Here's how the part is built. I have some questions about the finished solid (model axes, mm). A direction names the side the tool comes from. Round coordinates to 2 decimals unless told otherwise and drop trailing zeros. Order: outer loops, then holes, each group sorted by start corner. A loop starts at its lowest first (then second) coordinate and runs counter-clockwise, first axis right, second up. Notation, with made-up numbers: (56, -33) -> (99, -33) arc R29 ccw to (99, 1) -> close; hole circle Ø7 at (39, 67). An arc over 180 degrees is marked (long way). Answer in a Markdown table with one row per item.
```python
from build123d import *

# Parameters (mm, degrees)
SKETCH_W        = 30
SKETCH_H        = 30
PAD_DEPTH       = 3
POCKET_DEPTH    = 2.5
SKETCH002_R     = 1.725
POCKET001_DEPTH = 5
SKETCH003_R     = 1.225
PAD001_DEPTH    = 1.5


with BuildPart() as part:
    # Sketch → Pad (new body)
    with BuildSketch(Plane.XZ):
        Rectangle(SKETCH_W, SKETCH_H)
    extrude(amount=-PAD_DEPTH)

    # Sketch001 (on Face6 of Pad) → Pocket (cut)
    with BuildSketch(Plane(origin=(0, 3, 0), x_dir=(1, 0, 0), z_dir=(0, 1, 0))):
        Polygon((-11.616581, 7.2), (-8.383419, 7.2), (-6.766838, 10), (-8.383419, 12.8), (-11.616581, 12.8), (-13.233162, 10), align=None)
        Polygon((11.616581, 7.2), (13.233162, 10), (11.616581, 12.8), (8.383419, 12.8), (6.766838, 10), (8.383419, 7.2), align=None)
        Polygon((11.616581, -12.8), (13.233162, -10), (11.616581, -7.2), (8.383419, -7.2), (6.766838, -10), (8.383419, -12.8), align=None)
        Polygon((-8.383419, -7.2), (-11.616581, -7.2), (-13.233162, -10), (-11.616581, -12.8), (-8.383419, -12.8), (-6.766838, -10), align=None)
    extrude(amount=-POCKET_DEPTH, mode=Mode.SUBTRACT)

    # Sketch002 (on Face33 of Pocket) → Pocket001 (cut)
    with BuildSketch(Plane(origin=(0, 0.5, 0), x_dir=(1, 0, 0), z_dir=(0, 1, 0))):
        with Locations((-10, 10)):
            Circle(SKETCH002_R)
        with Locations((10, 10)):
            Circle(SKETCH002_R)
        with Locations((10, -10)):
            Circle(SKETCH002_R)
        with Locations((-10, -10)):
            Circle(SKETCH002_R)
    extrude(amount=-POCKET001_DEPTH, mode=Mode.SUBTRACT)

    # Sketch003 (on Face4 of Pocket001) → Pad001 (join)
    with BuildSketch(Plane.XZ):
        with Locations((4, -10)):
            Circle(SKETCH003_R)
        with Locations((-4, 10)):
            Circle(SKETCH003_R)
    extrude(amount=PAD001_DEPTH)


solid = part.part
```
1. Please list where these lines run through material, in increasing order: line 1 along Z through (x, y) = (10, 0.35) (3 decimals); line 2 along Z through (x, y) = (-12, 0.75).
Numbers:
| item | result |
|---|---|
| line 1 | z = -15 to -11.725, -8.275 to 8.275, 11.725 to 15 |
| line 2 | z = -15 to -12.14, -7.86 to 7.86, 12.14 to 15 |
2. Suppose I cut it at C-C on x = -4. Write out the boundary of the cut face in (y, z) (3 decimals).
Numbers:
| item | result |
|---|---|
| outline | (-1.5, 8.775) -> (0, 8.775) -> (0, -15) -> (3, -15) -> (3, 15) -> (0, 15) -> (0, 11.225) -> (-1.5, 11.225) -> close |
3. For faces 5 (the face through (-10.22, 0.25, 8.29)), 6 (the face through (-8.6, 0.5, 8.7)), which set-ups out of +Z, -Z, +X, -X, +Y, -Y let a thin tool reach every point of the face, with its end or its side?
Numbers:
| item | result |
|---|---|
| face 5 | +Y, -Y |
| face 6 | +Y |
4. For pin 1 Ø4 at (x, z) = (5.5, 6.5) entering from -Y; pin 2 Ø1.7 at (x, z) = (-10.5, 10.5) entering from +Y; pin 3 Ø4 at (x, z) = (10, -10) entering from +Y, each with a flat end and sliding along its axis, tell me the tip position at first contact or that it passes through.
Numbers:
| item | result |
|---|---|
| pin 1 | stops at y = 0 |
| pin 2 | passes through |
| pin 3 | stops at y = 0.5 |
5. Suppose I cut it at B-B on y = 2.1. Write out the boundary of the cut face in (x, z).
Numbers:
| item | result |
|---|---|
| outline | (-15, -15) -> (15, -15) -> (15, 15) -> (-15, 15) -> close; hole (-13.23, -10) -> (-11.62, -12.8) -> (-8.38, -12.8) -> (-6.77, -10) -> (-8.38, -7.2) -> (-11.62, -7.2) -> close; hole (-13.23, 10) -> (-11.62, 7.2) -> (-8.38, 7.2) -> (-6.77, 10) -> (-8.38, 12.8) -> (-11.62, 12.8) -> close; hole (6.77, -10) -> (8.38, -12.8) -> (11.62, -12.8) -> (13.23, -10) -> (11.62, -7.2) -> (8.38, -7.2) -> close; hole (6.77, 10) -> (8.38, 7.2) -> (11.62, 7.2) -> (13.23, 10) -> (11.62, 12.8) -> (8.38, 12.8) -> close |
6. We'd pull the mould along Z, two halves only. Please class faces 1 (the face through (0, 1, -15)), 2 (the face through (-4.97, -0.74, 9.25)), 3 (the face through (-7.564, 1.768, -11.38)), 4 (the face through (-12.436, 1.768, 11.38)): released by +Z, released by -Z, zero draft, split by the parting line, or undercut.
Numbers:
| item | result |
|---|---|
| face 1 | released by -Z |
| face 2 | split by the parting line |
| face 3 | undercut |
| face 4 | undercut |
7. Suppose I cut it at A-A on x = 10. Write out the boundary of the cut face in (y, z) (3 decimals).
Numbers:
| item | result |
|---|---|
| outline | (0, -15) -> (3, -15) -> (3, -12.8) -> (0.5, -12.8) -> (0.5, -11.725) -> (0, -11.725) -> close; (0, -8.275) -> (0.5, -8.275) -> (0.5, -7.2) -> (3, -7.2) -> (3, 7.2) -> (0.5, 7.2) -> (0.5, 8.275) -> (0, 8.275) -> close; (0, 11.725) -> (0.5, 11.725) -> (0.5, 12.8) -> (3, 12.8) -> (3, 15) -> (0, 15) -> close |
8. Suppose I cut it at D-D on z = -12.25. Write out the boundary of the cut face in (x, y), then the cut area to 3 significant figures.
Numbers:
| item | result |
|---|---|
| outline | (-15, 0) -> (15, 0) -> (15, 3) -> (11.93, 3) -> (11.93, 0.5) -> (8.07, 0.5) -> (8.07, 3) -> (-8.07, 3) -> (-8.07, 0.5) -> (-11.93, 0.5) -> (-11.93, 3) -> (-15, 3) -> close |
| area | 70.7 mm2 |
